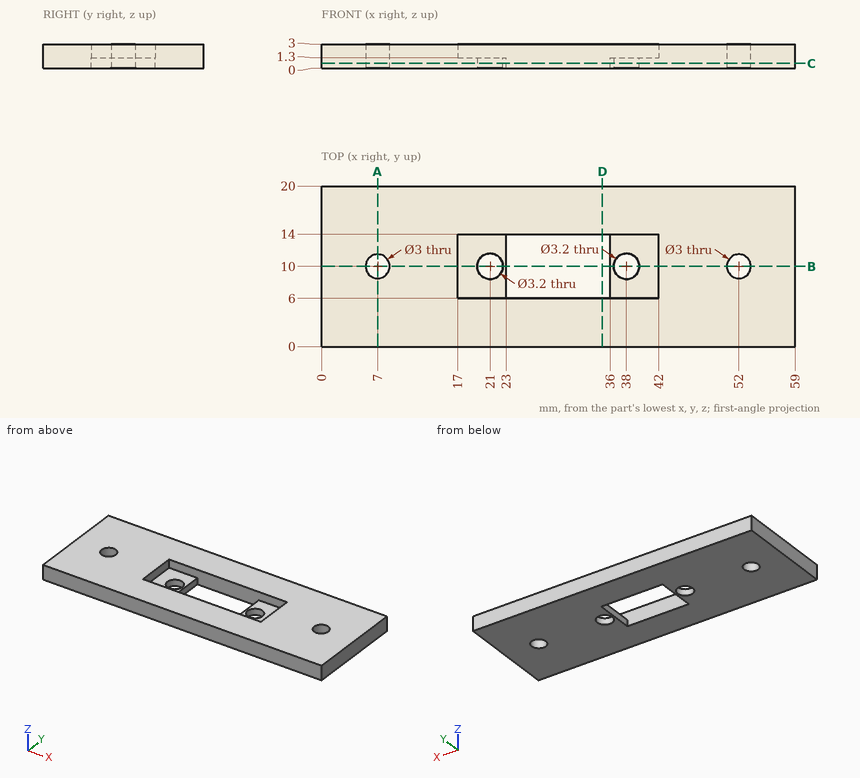
Drawing for the job (mm, zero at the part's lowest x, y, z). Give positions to 0.01 mm unless a question says otherwise; leave off trailing zeros. Order: outer loops, then holes, each group sorted by start corner. A loop starts at its lowest first (then second) coordinate and runs counter-clockwise, first axis right, second up. Notation, with made-up numbers: M -26,-13 L -10,-13 A15 cw -10,15 Z; hole C 72,40 d7. An arc over 180 degrees is marked long. Write item = value, one per line. Start each with the question number.
(1) Pin check, flat tips, straight feed: pin 1 Ø3 at (x, y) = (37.5, 8.5) entering from +Z; pin 2 Ø3 at (x, y) = (21, 10) entering from +Z; pin 3 Ø0.6 at (y, z) = (9.5, 1) entering from -X. Stop position of each tip, or through.
(2) Probe L1, parallel to Y at x = 7, z = 1.2; L2, parallel to Y at x = 26.5, z = 1.65; L3, parallel to X at y = 12.75, z = 0.1. List the from-to ranges inside material, lowest first. Write a range as [from, to].
(3) Slice it at C-C on z = 0.6. Write the cut outline in (x, y), plus the area to 3 significant figures.
(4) Slice it at A-A on x = 7. Write the cut outline in (y, z), plus the area to 3 significant figures.
(5) Slice it at D-D on x = 35. Write the cut outline in (y, z), plus the area to 3 significant figures.
(6) Slice it at B-B on y = 10. Write the cut outline in (x, z), plus the area to 3 significant figures.
Responses:
q1.pin_1 = 1.3
q1.pin_2 = through
q1.pin_3 = 0
q2.L1 = [0, 8.5], [11.5, 20]
q2.L2 = [0, 6], [14, 20]
q2.L3 = [0, 23], [36, 59]
q3.outline = M 0,0 L 59,0 L 59,20 L 0,20 Z; hole C 7,10 d3; hole C 21,10 d3.2; hole M 23,6 L 36,6 L 36,14 L 23,14 Z; hole C 38,10 d3.2; hole C 52,10 d3
q3.area = 1,050 mm2
q4.outline = M 0,0 L 8.5,0 L 8.5,3 L 0,3 Z; M 11.5,0 L 20,0 L 20,3 L 11.5,3 Z
q4.area = 51.0 mm2
q5.outline = M 0,0 L 6,0 L 6,3 L 0,3 Z; M 14,0 L 20,0 L 20,3 L 14,3 Z
q5.area = 36.0 mm2
q6.outline = M 0,0 L 5.5,0 L 5.5,3 L 0,3 Z; M 8.5,0 L 19.4,0 L 19.4,1.3 L 17,1.3 L 17,3 L 8.5,3 Z; M 22.6,0 L 23,0 L 23,1.3 L 22.6,1.3 Z; M 36,0 L 36.4,0 L 36.4,1.3 L 36,1.3 Z; M 39.6,0 L 50.5,0 L 50.5,3 L 42,3 L 42,1.3 L 39.6,1.3 Z; M 53.5,0 L 59,0 L 59,3 L 53.5,3 Z
q6.area = 91.3 mm2
